```python
from build123d import *

# Parameters (mm, degrees)
F0_W      = 40
F0_H      = 40
F0_W_2    = 34
F0_H_2    = 34
F1_DEPTH  = 380
F2_W      = 40
F2_H      = 40
F2_W_2    = 34
F2_H_2    = 34
F3_DEPTH  = 300
F4_W      = 40
F4_H      = 40
F4_W_2    = 34
F4_H_2    = 34
F5_DEPTH  = 380
F6_W      = 40
F6_H      = 40
F6_W_2    = 34
F6_H_2    = 34
F7_DEPTH  = 380
F8_W      = 40
F8_H      = 40
F8_W_2    = 34
F8_H_2    = 34
F9_DEPTH  = 300
F10_W     = 40
F10_H     = 40
F10_W_2   = 34
F10_H_2   = 34
F11_DEPTH = 300
F12_W     = 40
F12_H     = 40
F12_W_2   = 34
F12_H_2   = 34
F13_DEPTH = 300
F14_W     = 40
F14_H     = 40
F14_W_2   = 34
F14_H_2   = 34
F15_DEPTH = 300
F16_W     = 40
F16_H     = 40
F16_W_2   = 34
F16_H_2   = 34
F17_DEPTH = 380
F18_W     = 40
F18_H     = 40
F18_W_2   = 34
F18_H_2   = 33.7004394531
F19_DEPTH = 380
F20_W     = 40
F20_H     = 40
F20_W_2   = 34
F20_H_2   = 34
F21_DEPTH = 380
F22_DEPTH = 25
F23_W     = 40
F23_H     = 40
F23_W_2   = 34
F23_H_2   = 34
F24_DEPTH = 300
F25_W     = 40
F25_H     = 40
F25_W_2   = 34
F25_H_2   = 34
F26_DEPTH = 300
F27_W     = 40
F27_H     = 40
F27_W_2   = 34
F27_H_2   = 34
F28_DEPTH = 300
F29_W     = 40
F29_H     = 40
F29_W_2   = 34
F29_H_2   = 33.7004394531
F31_DEPTH = 300
F32_W     = 40
F32_H     = 40
F32_W_2   = 34
F32_H_2   = 34
F33_DEPTH = 300
F34_W     = 24
F34_H     = 24
F35_DEPTH = 300


with BuildPart() as f1:
    # F0 (on Top) → F1 (new body)
    with BuildSketch(Plane.XY):
        with Locations((-20, -20)):
            Rectangle(F0_W, F0_H)
        with Locations((-20, -20)):
            Rectangle(F0_W_2, F0_H_2, mode=Mode.SUBTRACT)
    extrude(amount=F1_DEPTH)

    # F2 (on face) → F3 (join)
    with BuildSketch(Plane.YZ):
        with Locations((-20, 20)):
            Rectangle(F2_W, F2_H)
        with Locations((-20, 20)):
            Rectangle(F2_W_2, F2_H_2, mode=Mode.SUBTRACT)
    extrude(amount=F3_DEPTH)

    # F4 (on face) → F5 (join)
    with BuildSketch(Plane(origin=(0, 0, 0), x_dir=(1, 0, 0), z_dir=(0, 0, -1))):
        with Locations((320, 20)):
            Rectangle(F4_W, F4_H)
        with Locations((320, 20)):
            Rectangle(F4_W_2, F4_H_2, mode=Mode.SUBTRACT)
    extrude(amount=-F5_DEPTH)

    # F6 (on face) → F7 (join)
    with BuildSketch(Plane(origin=(-40, 0, 0), x_dir=(0, -1, 0), z_dir=(-1, 0, 0))):
        with Locations((20, 400)):
            Rectangle(F6_W, F6_H)
        with Locations((20, 400)):
            Rectangle(F6_W_2, F6_H_2, mode=Mode.SUBTRACT)
    extrude(amount=-F7_DEPTH)

    # F8 (on face) → F9 (join)
    with BuildSketch(Plane(origin=(0, 0, 0), x_dir=(-1, 0, 0), z_dir=(0, 1, 0))):
        with Locations((20, 20)):
            Rectangle(F8_W, F8_H)
        with Locations((20, 20)):
            Rectangle(F8_W_2, F8_H_2, mode=Mode.SUBTRACT)
    extrude(amount=F9_DEPTH)

    # F10 (on face) → F11 (join)
    with BuildSketch(Plane(origin=(0, 0, 0), x_dir=(-1, 0, 0), z_dir=(0, 1, 0))):
        with Locations((-320, 20)):
            Rectangle(F10_W, F10_H)
        with Locations((-320, 20)):
            Rectangle(F10_W_2, F10_H_2, mode=Mode.SUBTRACT)
    extrude(amount=F11_DEPTH)

    # F12 (on face) → F13 (join)
    with BuildSketch(Plane(origin=(0, 0, 0), x_dir=(-1, 0, 0), z_dir=(0, 1, 0))):
        with Locations((-320, 400)):
            Rectangle(F12_W, F12_H)
        with Locations((-320, 400)):
            Rectangle(F12_W_2, F12_H_2, mode=Mode.SUBTRACT)
    extrude(amount=F13_DEPTH)

    # F14 (on face) → F15 (join)
    with BuildSketch(Plane(origin=(0, 0, 0), x_dir=(-1, 0, 0), z_dir=(0, 1, 0))):
        with Locations((20, 400)):
            Rectangle(F14_W, F14_H)
        with Locations((20, 400)):
            Rectangle(F14_W_2, F14_H_2, mode=Mode.SUBTRACT)
    extrude(amount=F15_DEPTH)

    # F16 (on face) → F17 (join)
    with BuildSketch(Plane(origin=(-40, 0, 0), x_dir=(0, -1, 0), z_dir=(-1, 0, 0))):
        with Locations((-320, 400)):
            Rectangle(F16_W, F16_H)
        with Locations((-320, 400)):
            Rectangle(F16_W_2, F16_H_2, mode=Mode.SUBTRACT)
    extrude(amount=-F17_DEPTH)

    # F18 (on face) → F19 (join)
    with BuildSketch(Plane(origin=(0, 0, 380), x_dir=(1, 0, 0), z_dir=(0, 0, -1))):
        with Locations((320, -320)):
            Rectangle(F18_W, F18_H)
        with Locations((320, -319.8502197266)):
            Rectangle(F18_W_2, F18_H_2, mode=Mode.SUBTRACT)
    extrude(amount=F19_DEPTH)

    # F20 (on face) → F21 (join)
    with BuildSketch(Plane(origin=(0, 0, 380), x_dir=(1, 0, 0), z_dir=(0, 0, -1))):
        with Locations((-20, -320)):
            Rectangle(F20_W, F20_H)
        with Locations((-20, -320)):
            Rectangle(F20_W_2, F20_H_2, mode=Mode.SUBTRACT)
    extrude(amount=F21_DEPTH)

    # F20 (on face) → F22 (join)
    with BuildSketch(Plane(origin=(0, 0, 380), x_dir=(1, 0, 0), z_dir=(0, 0, -1))):
        with Locations((-20, -320)):
            Rectangle(F20_W, F20_H)
        with Locations((-20, -320)):
            Rectangle(F20_W_2, F20_H_2, mode=Mode.SUBTRACT)
    extrude(amount=F22_DEPTH)

    # F23 (on face) → F24 (join)
    with BuildSketch(Plane(origin=(300, 0, 0), x_dir=(0, -1, 0), z_dir=(-1, 0, 0))):
        with Locations((-320, 20)):
            Rectangle(F23_W, F23_H)
        with Locations((-320, 20)):
            Rectangle(F23_W_2, F23_H_2, mode=Mode.SUBTRACT)
    extrude(amount=F24_DEPTH)

    # F25 (on face) → F26 (join)
    with BuildSketch(Plane(origin=(0, 0, 0), x_dir=(1, 0, 0), z_dir=(0, 0, -1))):
        with Locations((-20, 20)):
            Rectangle(F25_W, F25_H)
        with Locations((-20, 20)):
            Rectangle(F25_W_2, F25_H_2, mode=Mode.SUBTRACT)
    extrude(amount=F26_DEPTH)

    # F27 (on face) → F28 (join)
    with BuildSketch(Plane(origin=(0, 0, 0), x_dir=(1, 0, 0), z_dir=(0, 0, -1))):
        with Locations((320, 20)):
            Rectangle(F27_W, F27_H)
        with Locations((320, 20)):
            Rectangle(F27_W_2, F27_H_2, mode=Mode.SUBTRACT)
    extrude(amount=F28_DEPTH)

    # F29 (on face) → F31 (join)
    with BuildSketch(Plane(origin=(0, 0, 0), x_dir=(1, 0, 0), z_dir=(0, 0, -1))):
        with Locations((320, -320)):
            Rectangle(F29_W, F29_H)
        with Locations((320, -319.8502197266)):
            Rectangle(F29_W_2, F29_H_2, mode=Mode.SUBTRACT)
    extrude(amount=F31_DEPTH)

    # F32 (on face) → F33 (join)
    with BuildSketch(Plane(origin=(0, 0, 0), x_dir=(1, 0, 0), z_dir=(0, 0, -1))):
        with Locations((-20, -320)):
            Rectangle(F32_W, F32_H)
        with Locations((-20, -320)):
            Rectangle(F32_W_2, F32_H_2, mode=Mode.SUBTRACT)
    extrude(amount=F33_DEPTH)

    # F34 (on face) → F35 (join)
    with BuildSketch(Plane.YZ):
        Polygon((165, 35), (150, 35), (135, 35), (135, 5), (165, 5), align=None)
        with Locations((150, 20)):
            Rectangle(F34_W, F34_H, mode=Mode.SUBTRACT)
    extrude(amount=F35_DEPTH)


solid = f1.part
```
For this review, take the finished solid that the model builds, in its own axes (mm). A direction names the side the tool comes from. Give positions to 0.01 mm unless a question says otherwise; leave off trailing zeros. Answer as CSV lines item,"result".
1. For pin 1 (12 mm diameter, centred on x = 135, y = -12, fed in from -Z); pin 2 (12 mm diameter, centred on x = 124.5, y = 156, fed in from +Z), all flat-tipped, find the tip position at first contact; note any pin that passes through.
Findings:
pin 1,"stops at z = 0"
pin 2,"stops at z = 35"
2. Consider section A-A, the plane y = 233. Count the separate pieces of the cut face and the enclosed holes in it, then the cut area to 3 significant figures.
Findings:
separate pieces,"4"
enclosed holes,"4"
area,"1,780 mm2"
3. Wall thickness on line 1 (Z direction, x = 161.5, y = -10); line 2 (Y direction, x = 234.5, z = 23); line 3 (Y direction, x = 289, z = 38): over which ranges is each line inside the solid? List them lowest first.
Findings:
line 1,"z = 0 to 3, 37 to 40, 380 to 383, 417 to 420"
line 2,"y = -40 to -37, -3 to 0, 135 to 138, 162 to 165, 300 to 303, 337 to 340"
line 3,"y = -40 to 0, 300 to 340"
4. For faces 1 (the flat face through (148, 150, 35)), 2 (the flat face through (148, -3, 20)), 3 (the flat face through (147, -20, 417)), list the 3-axis set-ups (+Z, -Z, +X, -X, +Y, -Y) from which the entire face can be reached by the end or side of a thin tool; tool diameter is ignored.
Findings:
face 1,"+Z"
face 2,"none"
face 3,"+X, -X"
5. Draft analysis for pull direction Y (two halves, no side actions). For faces 4 (the flat face through (337.5, -20.3, -300)), 5 (the flat face through (148, 135, 20)), state which applies: +Y half, -Y half, draft (parallel to the pull), parting line (faces both ways), or undercut.
Findings:
face 4,"draft"
face 5,"undercut"
